Can you work these out from the drawing? Everything is in mm from the part's minimum corner. A direction names the side the tool comes from. Coordinates: 2 decimals unless noted, no trailing zeros. Write each loop counter-clockwise with the first axis right and the second up, starting at its lowest first coordinate (ties: lowest second). Pieces come first, ordered by that corner, then holes. Notation, with made-up numbers: M 38.25,55.25 L 68.25,55.25 A4 cw 68.25,61.25 Z; hole C -4,8.25 d1. An arc over 180 degrees is marked long. Write item = value, one per line.
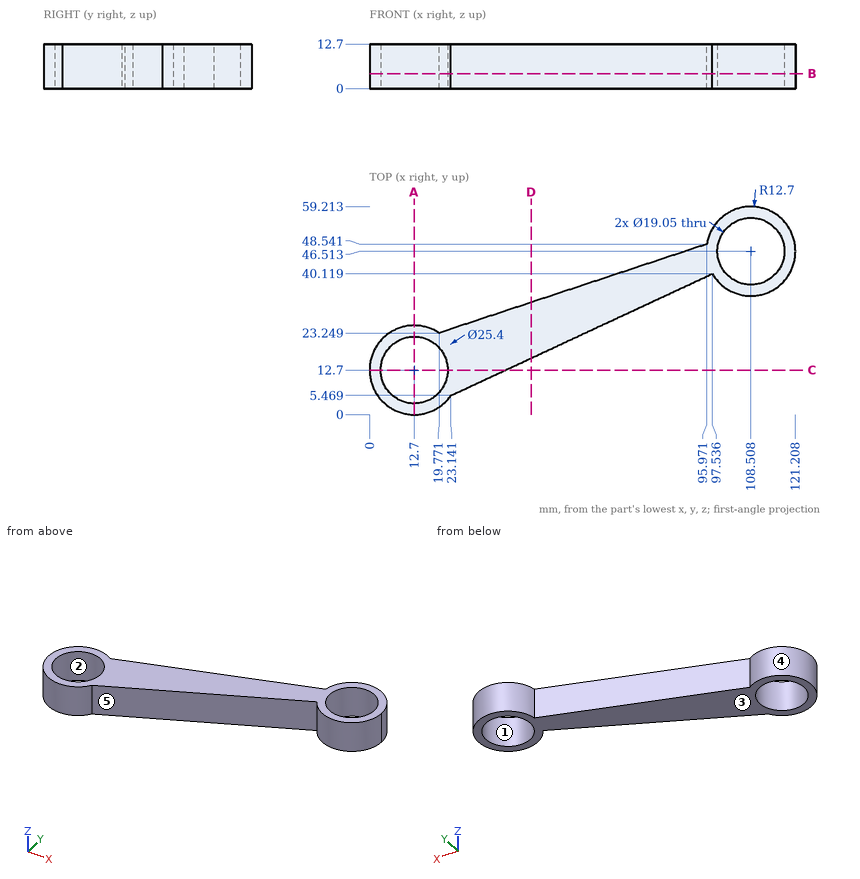
Item 1: Imagine slicing it at B-B (z = 4.25). State how many separate pieces and enclosed holes the cut face has, and give its area (3 significant figures).
Numbers:
separate_pieces = 1
enclosed_holes = 2
area = 1,450 mm²
Item 2: If I drill on line 1 along Y through (x, z) = (12.7, 4) (1 decimal); line 2 along X through (y, z) = (18.5, 1.25) (1 decimal); line 3 along Y through (x, z) = (113, 3) (1 decimal), over which ranges is the centre line in solid material (lowest first)?
Numbers:
line_1 = 0 to 3.2, 22.2 to 25.4
line_2 = 1.4 to 5.1, 20.3 to 51.1
line_3 = 34.6 to 38.1, 54.9 to 58.4
Item 3: I'm going to push flat-ended pins straight in: P1, Ø15, axis at x = 108.51, y = 46.51, coming from the +Z side; P2, Ø4, axis at y = 29, z = 7.5, coming from the +X side (1 decimal); P3, Ø2, axis at x = 81.5, z = 11, coming from the -Y side (1 decimal). Where does each tip first touch, or does it pass through?
Numbers:
P1 = through
P2 = 78
P3 = 32.2
Item 4: Imagine slicing it at A-A (x = 12.7). Write out the boundary of the cut face in (y, z) (1 decimal).
Numbers:
outline = M 0,0 L 3.2,0 L 3.2,12.7 L 0,12.7 Z; M 22.2,0 L 25.4,0 L 25.4,12.7 L 22.2,12.7 Z
Item 5: For the marked faces 4 and 5, which set-ups out of +Z, -Z, +X, -X, +Y, -Y let a thin tool reach every point of the face, with its end or its side?
Numbers:
face_4 = +Z, -Z
face_5 = +Z, -Z, -Y
Item 6: Imagine slicing it at D-D (x = 46). Write out the boundary of the cut face in (y, z) (1 decimal), and give its area (3 significant figures).
Numbers:
outline = M 16.1,0 L 32,0 L 32,12.7 L 16.1,12.7 Z
area = 201 mm²
Item 7: If we mould it in two halves opening along X, with no side actions, what happens to the marked faces 1, 2 and 3? For each: pulls with the +X half, pulls with the -X half, needs draft (parallel to the pull), parting line crosses it, or undercut.
Numbers:
face_1 = undercut
face_2 = undercut
face_3 = needs draft
Item 8: Imagine slicing it at C-C (y = 12.7). Write out the boundary of the cut face in (x, z) (1 decimal).
Numbers:
outline = M 0,0 L 3.2,0 L 3.2,12.7 L 0,12.7 Z; M 22.2,0 L 38.7,0 L 38.7,12.7 L 22.2,12.7 Z
